The model under review builds one solid part; all positions refer to its coordinate system, in mm. A direction names the side the tool comes from. Give positions to 0.01 mm unless a question says otherwise; leave off trailing zeros. Write each loop counter-clockwise with the first axis right and the second up, starting at its lowest first coordinate (ties: lowest second). Pieces come first, ordered by that corner, then holes. Notation, with made-up numbers: (25, 10.5) - (81, 10.5) arc R11 ccw to (81, 20.5) - close; hole circle Ø1 at (-26.75, 70). An arc over 180 degrees is marked (long way). One line per question, with ' | ' between items. Start each with the question number.
```python
from build123d import *

# Parameters (mm, degrees)
F1_DEPTH = 7.62
F2_T     = -2.54
F4_DEPTH = 5.08


with BuildPart() as f1:
    # F0 (on Top) → F1 (new body)
    with BuildSketch(Plane.XY):
        Polygon((32.0682525635, -14.3153322861), (3.4442073984, 39.2894335091), (-27.6627708226, 39.2894335091), (-27.6627708226, -44.8362566531), (60.85267663, -44.8362566531), (81.4588740468, -33.4062539041), (81.4588740468, -20.4415936023), (32.0682525635, -20.4415936023), align=None)
    extrude(amount=F1_DEPTH)

    # F2
    f2_openings = [f1.faces().sort_by_distance(p)[0] for p in [
        (9.989967, -12.135941, 7.62),
    ]]
    offset(amount=F2_T, openings=f2_openings, kind=Kind.INTERSECTION)

    # F3 (on face) → F4 (join)
    with BuildSketch(Plane.XY.offset(2.54)):
        Polygon((25.0375904143, -18.7208298594), (0, 31.1848036945), (-19.5555072278, 31.1848036945), (-19.5555072278, -38.3611097932), (59.4885759056, -38.3611097932), (74.9432295561, -27.8970263898), (74.9432295561, -27.4460842204), (25.0375904143, -27.4460842204), align=None)
    extrude(amount=F4_DEPTH)


solid = f1.part
```
Item 1: Machinability: for faces 1 (the flat face through (55, -22.982, 5)), 2 (the flat face through (-12, 39.289, 4)), which of the approach directions +Z, -Z, +X, -X, +Y, -Y give a long, thin tool a straight path to every point of the face, cutting with its end or side? Answer none if there is none.
Item 2: Take a section at B-B (x = 39). Give the boundary of the cut face in (y, z), plus the area to 3 significant figures.
Item 3: Take a section at C-C (y = 23). Give the boundary of the cut face in (x, z), plus the area to 3 significant figures.
Item 4: For probe 1 along Y at (x, z) = (52, 6); probe 2 along Y at (x, z) = (-19, 6.5); probe 3 along X at (y, z) = (0.5, 4.75), list the stretches that pass through material, from the lowest coordinate up.
Item 5: Take a section at A-A (z = 5). Give the boundary of the cut face in (x, y).
Item 6: Clearance check with flat-ended pins moving along their axes: P1, Ø1, axis at y = -1, z = 1, coming from the +X side; P2, Ø2, axis at y = -17, z = 5, coming from the +X side; P3, Ø4, axis at y = 11.5, z = 2, coming from the +X side. State where each tip first meets the part, or that it passes through.
Item 7: The part is to be moulded in two halves that separate along Y. For faces 3 (the flat face through (67.11, -33.2, 5.04)), 4 (the flat face through (32.068, -17, 4)), 5 (the flat face through (17.957, 12.112, 3.757)), say which applies: +Y half, -Y half, draft (parallel to the pull), parting line (faces both ways), or undercut.
Check sheet entries:
1) face 1: +Z | face 2: +Z, -Z, +X, -X, +Y
2) outline: (-44.84, 0) - (-20.44, 0) - (-20.44, 7.62) - (-22.98, 7.62) - (-22.98, 2.54) - (-27.45, 2.54) - (-27.45, 7.62) - (-38.36, 7.62) - (-38.36, 2.54) - (-42.3, 2.54) - (-42.3, 7.62) - (-44.84, 7.62) - close | area: 143 mm^2
3) outline: (-27.66, 0) - (12.14, 0) - (12.14, 7.62) - (9.26, 7.62) - (9.26, 2.54) - (4.11, 2.54) - (4.11, 7.62) - (-19.56, 7.62) - (-19.56, 2.54) - (-25.12, 2.54) - (-25.12, 7.62) - (-27.66, 7.62) - close | area: 249 mm^2
4) probe 1: y = -44.84 to -42.3, -38.36 to -27.45, -22.98 to -20.44 | probe 2: y = -44.84 to -42.3, -38.36 to 31.18, 36.75 to 39.29 | probe 3: x = -27.66 to -25.12, -19.56 to 15.39, 21.28 to 24.16
5) outline: (-27.66, -44.84) - (60.85, -44.84) - (81.46, -33.41) - (81.46, -20.44) - (32.07, -20.44) - (32.07, -14.32) - (3.44, 39.29) - (-27.66, 39.29) - close; (-19.56, -38.36) - (59.49, -38.36) - (74.94, -27.9) - (74.94, -27.45) - (25.04, -27.45) - (25.04, -18.72) - (0, 31.18) - (-19.56, 31.18) - close; hole (-25.12, -42.3) - (60.2, -42.3) - (78.92, -31.91) - (78.92, -22.98) - (29.53, -22.98) - (29.53, -14.95) - (1.92, 36.75) - (-25.12, 36.75) - close
6) P1: stops at x = 25.23 | P2: stops at x = 32.07 | P3: stops at x = 19.35
7) face 3: undercut | face 4: draft | face 5: +Y half
